Part model, mm, in its own coordinate system. Face numbers are marked on the shaded views. A direction names the side the tool comes from. Round coordinates to 2 decimals unless told otherwise and drop trailing zeros. Write each loop counter-clockwise with the first axis right and the second up, starting at its lowest first coordinate (ties: lowest second). Pieces come first, ordered by that corner, then holes.
1) Which spindle directions (+Z, -Z, +X, -X, +Y, -Y) get a long thin tool onto all of the face, cutting with end or side? Do the marked faces 1 and 2. Say none if no direction does.
2) Saw through at C-C on y = 52. Write the cut outline in (x, z).
3) Saw through at B-B on z = 3.25. Write the cut outline in (x, y).
4) Saw through at A-A on y = 72.5. Write the cut outline in (x, z).
5) Drill centre lines: L1, parallel to Y at x = -10, z = 1.7; L2, parallel to Y at x = -5.75, z = 10.5; L3, parallel to X at y = 63.45, z = 9. Where is each one in solid material? Low to high.
6) Pull direction Z, two halves, no side cores. Call the marked faces 3, 4 and 5: +Z half, -Z half, draft (parallel to the pull), parting line (faces both ways), or undercut.
7) Saw through at D-D on z = 13. Write the cut outline in (x, y).
8) Flat gauge pins, fed straight in: pin 1 (2.5 mm diameter, centred on y = 18, z = 9.5, fed in from +X); pin 2 (9.5 mm diameter, centred on x = -10, y = 7.5, fed in from +Z); pin 3 (5 mm diameter, centred on x = -10, z = 9, fed in from -Y); pin 4 (2.5 mm diameter, centred on x = -10, z = 9, fed in from +Y). Where does each tip first touch, or does it go through?
```python
from build123d import *

# Parameters (mm, degrees)
ESQUISSE1_W             = 20
ESQUISSE1_H             = 80
BOSS_EXTRU_1_DEPTH      = 4
ESQUISSE2_W             = 10
ESQUISSE2_H             = 5
BOSS_EXTRU_2_DEPTH      = 10
ESQUISSE3_R             = 2.25
ENL_V_MAT_EXTRU_1_DEPTH = 66
CONG_1_R                = 2
CONG_2_R                = 4
ESQUISSE4_R             = 3
ENL_V_MAT_EXTRU_2_DEPTH = 5


with BuildPart() as part:
    # Esquisse1 → Boss.-Extru.1 (new body)
    with BuildSketch(Plane.XY):
        with Locations((-10, 40)):
            Rectangle(ESQUISSE1_W, ESQUISSE1_H)
    extrude(amount=BOSS_EXTRU_1_DEPTH)

    # Esquisse2 → Boss.-Extru.2 (add)
    with BuildSketch(Plane.XY.offset(4)):
        with Locations((-10, 62.5)):
            Rectangle(ESQUISSE2_W, ESQUISSE2_H)
        with Locations((-10, 52.5)):
            Rectangle(ESQUISSE2_W, ESQUISSE2_H)
        with Locations((-10, 27.5)):
            Rectangle(ESQUISSE2_W, ESQUISSE2_H)
        with Locations((-10, 17.5)):
            Rectangle(ESQUISSE2_W, ESQUISSE2_H)
    extrude(amount=BOSS_EXTRU_2_DEPTH)

    # Esquisse3 → Enlèv. mat.-Extru.1 (cut, through all)
    with BuildSketch(Plane.XZ.offset(-15)):
        with Locations(Location((-10, 9, 0), (0, 0, 270))):  # turned: the seam where the file's is
            Circle(ESQUISSE3_R)
    extrude(amount=-ENL_V_MAT_EXTRU_1_DEPTH, mode=Mode.SUBTRACT)

    # Congé1
    cong_1_edges = [part.edges().sort_by_distance(p)[0] for p in [
        (-15, 62.5, 14),
        (-5, 62.5, 14),
        (-15, 52.5, 14),
        (-5, 52.5, 14),
        (-15, 27.5, 14),
        (-5, 27.5, 14),
        (-15, 17.5, 14),
        (-5, 17.5, 14),
    ]]
    fillet(cong_1_edges, radius=CONG_1_R)

    # Congé2
    cong_2_edges = [part.edges().sort_by_distance(p)[0] for p in [
        (-20, 80, 2),
        (0, 80, 2),
        (0, 0, 2),
        (-20, 0, 2),
    ]]
    fillet(cong_2_edges, radius=CONG_2_R)

    # Esquisse4 → Enlèv. mat.-Extru.2 (cut, through all)
    with BuildSketch(Plane.XY.offset(4)):
        with Locations((-10, 7.5)):
            Circle(ESQUISSE4_R)
        with Locations((-10, 72.5)):
            Circle(ESQUISSE4_R)
        with Locations((-10, 40)):
            Circle(ESQUISSE4_R)
    extrude(amount=-ENL_V_MAT_EXTRU_2_DEPTH, mode=Mode.SUBTRACT)


solid = part.part
```
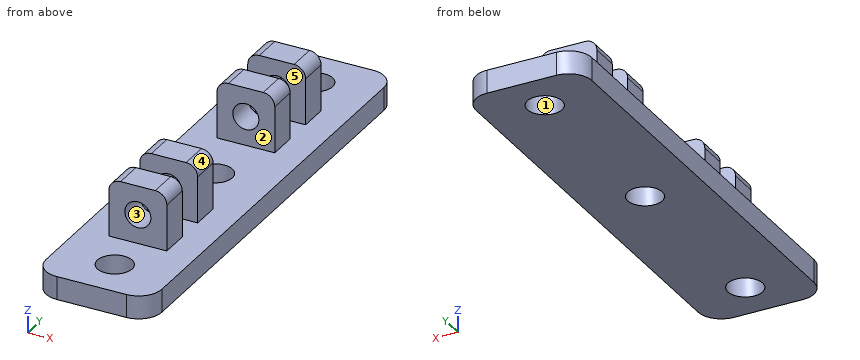
Completed:
1. face 1: +Z, -Z
1. face 2: +Z, +X, -X
2. outline: (-20, 0) - (0, 0) - (0, 4) - (-5, 4) - (-5, 12) arc R2 ccw to (-7, 14) - (-13, 14) arc R2 ccw to (-15, 12) - (-15, 4) - (-20, 4) - close; hole circle Ø4.5 at (-10, 9)
3. outline: (-20, 4) arc R4 ccw to (-16, 0) - (-4, 0) arc R4 ccw to (0, 4) - (0, 76) arc R4 ccw to (-4, 80) - (-16, 80) arc R4 ccw to (-20, 76) - close; hole circle Ø6 at (-10, 7.5); hole circle Ø6 at (-10, 40); hole circle Ø6 at (-10, 72.5)
4. outline: (-20, 0) - (-13, 0) - (-13, 4) - (-20, 4) - close; (-7, 0) - (0, 0) - (0, 4) - (-7, 4) - close
5. L1: y = 0 to 4.5, 10.5 to 37, 43 to 69.5, 75.5 to 80
5. L2: y = 15 to 20, 25 to 30, 50 to 55, 60 to 65
5. L3: x = -15 to -12.25, -7.75 to -5
6. face 3: undercut
6. face 4: +Z half
6. face 5: draft
7. outline: (-14.73, 15) - (-5.27, 15) - (-5.27, 20) - (-14.73, 20) - close; (-14.73, 25) - (-5.27, 25) - (-5.27, 30) - (-14.73, 30) - close; (-14.73, 50) - (-5.27, 50) - (-5.27, 55) - (-14.73, 55) - close; (-14.73, 60) - (-5.27, 60) - (-5.27, 65) - (-14.73, 65) - close
8. pin 1: stops at x = -5
8. pin 2: stops at z = 4
8. pin 3: stops at y = 15
8. pin 4: passes through
